from build123d import *

# Parameters (mm, degrees)
BOSS_EXTRUDE1_DEPTH = 7.5
SKETCH2_R           = 12.5
BOSS_EXTRUDE2_DEPTH = 15
SKETCH3_R           = 30
CUT_EXTRUDE1_DEPTH  = 15
BOSS_EXTRUDE3_DEPTH = 2.5
SKETCH5_R           = 10
CUT_EXTRUDE2_DEPTH  = 102.261018189
CHAMFER1_SIZE       = 1
CHAMFER2_SIZE       = 8
CHAMFER3_SIZE       = 2


with BuildPart() as part:
    # Sketch1 → Boss-Extrude1 (new, symmetric)
    with BuildSketch(Plane(origin=(0, 0, 0), x_dir=(1, 0, 0), z_dir=(0, 1, 0))):
        Polygon((-40, 0), (40, 0), (12.5, 75.555629035), (-12.5, 75.555629035), align=None)
    extrude(amount=BOSS_EXTRUDE1_DEPTH, both=True)

    # Sketch2 → Boss-Extrude2 (add, symmetric)
    with BuildSketch(Plane(origin=(0, 0, 0), x_dir=(1, 0, 0), z_dir=(0, 1, 0))):
        with Locations(Location((0, 75.555629035, 0), (0, 0, 270))):
            Circle(SKETCH2_R)
    extrude(amount=BOSS_EXTRUDE2_DEPTH, both=True)

    # Sketch3 → Cut-Extrude1 (cut, symmetric)
    with BuildSketch(Plane(origin=(0, 0, 0), x_dir=(1, 0, 0), z_dir=(0, 1, 0))):
        Circle(SKETCH3_R)
    extrude(amount=CUT_EXTRUDE1_DEPTH, both=True, mode=Mode.SUBTRACT)

    # Sketch4 → Boss-Extrude3 (add, symmetric)
    with BuildSketch(Plane(origin=(0, 0, 0), x_dir=(1, 0, 0), z_dir=(0, 1, 0))):
        with BuildLine():
            Line((-30, 0), (-25, 0))
            ThreePointArc((-25, 0), (0, 25), (25, 0))
            Line((25, 0), (30, 0))
            ThreePointArc((30, 0), (0, 30), (-30, 0))
        make_face()
    extrude(amount=BOSS_EXTRUDE3_DEPTH, both=True)

    # Sketch5 → Cut-Extrude2 (cut, through all)
    with BuildSketch(Plane(origin=(0, 15, 0), x_dir=(1, 0, 0), z_dir=(0, 1, 0))):
        with Locations(Location((0, 75.555629035, 0), (0, 0, 270))):
            Circle(SKETCH5_R)
    extrude(amount=-CUT_EXTRUDE2_DEPTH, mode=Mode.SUBTRACT)

    # Chamfer1
    chamfer1_edges = [part.edges().sort_by_distance(p)[0] for p in [
        (0, -7.5, -30),
        (0, 7.5, -30),
        (0, -2.5, -25),
        (0, 2.5, -25),
    ]]
    chamfer(chamfer1_edges, length=CHAMFER1_SIZE)

    # Chamfer2
    chamfer2_edges = [part.edges().sort_by_distance(p)[0] for p in [
        (40, 0, 0),
        (-40, 0, 0),
    ]]
    chamfer(chamfer2_edges, length=CHAMFER2_SIZE)

    # Chamfer3
    chamfer3_edges = [part.edges().sort_by_distance(p)[0] for p in [
        (-24.881919427, 7.5, -41.536585001),
        (-24.881919427, -7.5, -41.536585001),
        (24.881919427, -7.5, -41.536585001),
        (24.881919427, 7.5, -41.536585001),
    ]]
    chamfer(chamfer3_edges, length=CHAMFER3_SIZE)


solid = part.part
Work out the finished part from the listing and answer in its coordinate system (mm). A direction names the side the tool comes from. Round coordinates to 2 decimals unless told otherwise and drop trailing zeros. Write each loop counter-clockwise with the first axis right and the second up, starting at its lowest first coordinate (ties: lowest second). Pieces come first, ordered by that corner, then holes. Notation, with made-up numbers: (81, -34) - (104, -34) arc R15 cw to (104, -28) - close; hole circle Ø4 at (-11, 16). An arc over 180 degrees is marked (long way). Answer in a Markdown table with one row per item. Add a question column.
1. The mould has two halves that part along X. Classify faces 4 (the flat face through (-0.1, 2.5, -26.2)), 5 (the flat face through (-1, 7.5, -36)), 6 (the flat face through (-24.018, -6.486, -41.027)), 7 (the cylindrical face through (0.66, -4.472, -29.993)): +X half, -X half, draft (parallel to the pull), parting line (faces both ways), or undercut.
2. A cutting plane is placed at A-A, the plane x = 0. Determine the outline of the cut face in (y, z), and give its area (3 significant figures).
3. Given pin 1 (1.5 mm diameter, centred on y = -1.5, z = -28, fed in from -X); pin 2 (15 mm diameter, centred on x = 7.5, z = -13.5, fed in from -Y); pin 3 (1.5 mm diameter, centred on x = 6.5, z = -42, fed in from +Y); pin 4 (6 mm diameter, centred on x = 11.5, y = -8, fed in from +Z), each flat-ended and moving along its own axis, determine where each tip first touches the part or whether it passes through.
4. For faces 1 (the cylindrical face through (0.66, 4.528, -29.993)), 2 (the flat face through (-34.67, 0.11, -3.81)), 3 (the cylindrical face through (0.55, 0.21, -88.044)), determine the directions among +Z, -Z, +X, -X, +Y, -Y from which every point of the face is accessible in a straight line to the end or side of a thin tool.
5. A cutting plane is placed at B-B, the plane y = -4.5. Determine the outline of the cut face in (x, z).
6. Find the intervals of material crossed by line 1 along X through (y, z) = (7.5, -75); line 2 along Y through (x, z) = (12.5, -25.5); line 3 along Z through (x, y) = (6, -8.5), in increasing order. Write a range as from..to.
Worked out:
| question | item | result |
|---|---|---|
| 1 | face 4 | undercut |
| 1 | face 5 | draft |
| 1 | face 6 | -X half |
| 1 | face 7 | undercut |
| 2 | outline | (-15, -88.06) - (15, -88.06) - (15, -85.56) - (-15, -85.56) - close; (-15, -65.56) - (15, -65.56) - (15, -63.06) - (7.5, -63.06) - (7.5, -31) - (6.5, -30) - (2.5, -30) - (2.5, -26) - (1.5, -25) - (-1.5, -25) - (-2.5, -26) - (-2.5, -30) - (-6.5, -30) - (-7.5, -31) - (-7.5, -63.06) - (-15, -63.06) - close |
| 2 | area | 669 mm^2 |
| 3 | pin 1 | x = -30.08 |
| 3 | pin 2 | through |
| 3 | pin 3 | y = 7.5 |
| 3 | pin 4 | z = -26.48 |
| 4 | face 1 | +Z, +Y |
| 4 | face 2 | +Z, -X, +Y, -Y |
| 4 | face 3 | none |
| 5 | outline | (-37.26, -7.52) - (-12.5, -75.56) arc R12.5 ccw to (12.5, -75.56) - (37.26, -7.52) - (32, 0) - (30, 0) arc R30 cw to (-30, 0) - (-32, 0) - close; hole circle Ø20 at (0, -75.56) |
| 6 | line 1 | -12.49..-9.98, 9.98..12.49 |
| 6 | line 2 | -2.5..2.5 |
| 6 | line 3 | -86.52..-83.56, -67.56..-64.59 |
